The listing builds one solid part. Answer for the finished solid, in the listing's coordinates (mm). A direction names the side the tool comes from. Give positions to 0.01 mm unless a question says otherwise; leave off trailing zeros. Write each loop counter-clockwise with the first axis right and the second up, starting at its lowest first coordinate (ties: lowest second). Pieces come first, ordered by that corner, then holes. Notation, with made-up numbers: M 13,29 L 35,29 A33 cw 35,60 Z; hole C -13,22.25 d3. An arc over 180 degrees is marked long. Return JSON: item names as keys, results as strings.
from build123d import *

# Parameters (mm, degrees)
PAD001_START    = 6
SKETCH007_R     = 9
PAD001_DEPTH    = 6
SKETCH008_R     = 1.7
HOLE001_DEPTH   = 6.001
POCKET006_START = -5
SKETCH009_R     = 3.8
POCKET006_DEPTH = 95
SKETCH010_R     = 2.1
POCKET007_DEPTH = 58.307787
CHAMFER_SIZE    = 0.5


with BuildPart() as part:
    # Sketch007 → Pad001 (new body)
    with BuildSketch(Plane.XY.offset(PAD001_START)):
        Circle(SKETCH007_R)
    extrude(amount=PAD001_DEPTH)

    # Sketch008 (on Face3 of Pad001) → Hole001 (cut, through all)
    with BuildSketch(Plane.XY.offset(12)):
        with Locations((0, 5)):
            Circle(SKETCH008_R)
    extrude(amount=-HOLE001_DEPTH, mode=Mode.SUBTRACT)

    # Sketch009 (on Face3 of Hole001) → Pocket006 (cut)
    with BuildSketch(Plane.XY.offset(12).offset(POCKET006_START)):
        with Locations((0, 5)):
            Circle(SKETCH009_R)
    extrude(amount=-POCKET006_DEPTH, mode=Mode.SUBTRACT)

    # Sketch010 (on Face3 of Pocket006) → Pocket007 (cut, through all)
    with BuildSketch(Plane.XY.offset(12)):
        with Locations((-4, -3.5)):
            Circle(SKETCH010_R)
    pocket007 = extrude(amount=-POCKET007_DEPTH, mode=Mode.SUBTRACT)

    # Mirrored001: Pocket007 across YZ
    add(pocket007.mirror(Plane.YZ), mode=Mode.SUBTRACT)

    # Chamfer
    chamfer_edges = [part.edges().sort_by_distance(p)[0] for p in [
        (6.1, -3.5, 12),
        (-6.1, -3.5, 12),
    ]]
    chamfer(chamfer_edges, length=CHAMFER_SIZE)


solid = part.part
Item 1: A cutting plane is placed at B-B, the plane y = -3.5. Write down the section's boundary in (x, z).
Geometry results:
{"outline": "M -8.29,6 L -6.1,6 L -6.1,11.5 L -6.6,12 L -8.29,12 Z; M -1.9,6 L 1.9,6 L 1.9,11.5 L 1.4,12 L -1.4,12 L -1.9,11.5 Z; M 6.1,6 L 8.29,6 L 8.29,12 L 6.6,12 L 6.1,11.5 Z"}
Item 2: A cutting plane is placed at A-A, the plane x = 0. Write down the section's boundary in (y, z), plus the area to 3 significant figures.
Geometry results:
{"outline": "M -9,6 L 1.2,6 L 1.2,7 L 3.3,7 L 3.3,12 L -9,12 Z; M 6.7,7 L 8.8,7 L 8.8,6 L 9,6 L 9,12 L 6.7,12 Z", "area": "83.4 mm2"}
Item 3: Determine the mould class of faces 1 (the cylindrical face through (4.46, -5.55, 8.79)), 2 (the flat face through (0, -2, 6)), 3 (the cylindrical face through (-1.172, 8.923, 8.958)) for opening direction X: +X half, -X half, draft (parallel to the pull), parting line (faces both ways), or undercut.
Geometry results:
{"face 1": "undercut", "face 2": "draft", "face 3": "parting line"}
Item 4: A cutting plane is placed at D-D, the plane y = 4.75. Write down the section's boundary in (x, z).
Geometry results:
{"outline": "M -7.64,6 L -3.79,6 L -3.79,7 L -1.68,7 L -1.68,12 L -7.64,12 Z; M 1.68,7 L 3.79,7 L 3.79,6 L 7.64,6 L 7.64,12 L 1.68,12 Z"}
Item 5: A cutting plane is placed at C-C, the plane z = 6.45. Write down the section's boundary in (x, y), plus the area to 3 significant figures.
Geometry results:
{"outline": "C 0,0 d18; hole C -4,-3.5 d4.2; hole C 0,5 d7.6; hole C 4,-3.5 d4.2", "area": "181 mm2"}
Item 6: Given pin 1 Ø1.5 at (y, z) = (2, 10) entering from +X; pin 2 Ø3 at (x, z) = (-4, 10) entering from -Y; pin 3 Ø2 at (y, z) = (-2.5, 7.5) entering from -X, each flat-ended and moving along its own axis, determine where each tip first touches the part or whether it passes through.
Geometry results:
{"pin 1": "stops at x = 8.91", "pin 2": "stops at y = -8.65", "pin 3": "stops at x = -8.87"}
Item 7: Find the intervals of material crossed by line 1 (Y direction, x = 0, z = 6.45); line 2 (X direction, y = -4, z = 11.1); line 3 (Y direction, x = 0, z = 10.6), in increasing order.
Geometry results:
{"line 1": "y = -9 to 1.2, 8.8 to 9", "line 2": "x = -8.06 to -6.04, -1.96 to 1.96, 6.04 to 8.06", "line 3": "y = -9 to 3.3, 6.7 to 9"}
Item 8: Which of the six approach directions +Z, -Z, +X, -X, +Y, -Y give full straight-line access (tool end or side, diameter ignored) to faces 4 (the flat face through (0, 0, 12)), 5 (the cylindrical face through (3.625, 6.141, 6.507))?
Geometry results:
{"face 4": "+Z, +X, -X, +Y, -Y", "face 5": "-Z"}
